from build123d import *

# Parameters (mm, degrees)
F1_DEPTH = 23
F3_DEPTH = 21
F4_R     = 12.5
F4_R_2   = 1.75
F5_DEPTH = 22.001


with BuildPart() as f1:
    # F0 (on Right) → F1 (new body, symmetric)
    with BuildSketch(Plane.YZ):
        Polygon((2, 44), (0, 44), (0, 0), (22, 0), (22, 2), align=None)
    extrude(amount=F1_DEPTH, both=True)

    # F2 (on Right) → F3 (cut, symmetric)
    with BuildSketch(Plane.YZ):
        Polygon((2, 2), (22, 2), (2, 44), align=None)
    extrude(amount=F3_DEPTH, both=True, mode=Mode.SUBTRACT)

    # F4 (on face) → F5 (cut, through all)
    with BuildSketch(Plane.XZ):
        with Locations((0, 23)):
            Circle(F4_R)
        with Locations((-15.5, 38.5)):
            Circle(F4_R_2)
        with Locations((-15.5, 7.5)):
            Circle(F4_R_2)
        with Locations((15.5, 38.5)):
            Circle(F4_R_2)
        with Locations((15.5, 7.5)):
            Circle(F4_R_2)
    extrude(amount=-F5_DEPTH, mode=Mode.SUBTRACT)


solid = f1.part
Input: part model. Units: mm. Frame: model coordinates. A direction names the side the tool comes from. Give positions to 0.01 mm unless a question says otherwise; leave off trailing zeros. Loops run counter-clockwise (first coordinate to the right, second up) from the corner with the lowest first, then second, coordinate; pieces in that order, holes last. Notation, with made-up numbers: (4, 12) -> (27, 12) arc R19 cw to (27, 39) -> close; hole circle Ø10 at (-14, -30). An arc over 180 degrees is marked (long way). Answer as a JSON object with one key per item and string values. Group by question number.
Item 1: Pull-direction query (X, two-part tool) for faces 3 (the flat face through (-22, 12, 23)), 4 (the flat face through (23, 8, 17)), 5 (the flat face through (0, 12, 2)); classes: released by +X, released by -X, zero draft, split by the parting line, or undercut.
Item 2: Cut plane D-D, the plane z = 26. Return the cut outline in (x, y), and give its area (3 significant figures).
Item 3: Cut plane B-B, the plane z = 38.5. Return the cut outline in (x, y), and give its area (3 significant figures).
Item 4: Cut plane C-C, the plane y = 16. Return the cut outline in (x, z).
Item 5: Cut plane A-A, the plane x = 0. Return the cut outline in (y, z), and give its area (3 significant figures).
Item 6: Reachability of faces 1 (the flat face through (21, 7, 14)), 2 (the flat face through (-10, 0, 13)) from +Z, -Z, +X, -X, +Y, -Y: full face, straight path, thin tool, end or side. Return the list, or none.
Item 7: Line query: probe 1 along Z at (x, y) = (15.5, 0.5); probe 2 along X at (y, z) = (11.5, 20.5); probe 3 along Z at (x, y) = (-4, 4.25). Output: solid intervals per line, ascending.
Item 8: Pin query (flat end, axial travel): P1, Ø3, axis at x = -14, z = 23.5, coming from the +Y side. Return the tip coordinate at first contact, or that it passes through.
Checks:
{
 "1": {"face 3": "zero draft", "face 4": "released by +X", "face 5": "undercut"},
 "2": {"outline": "(-23, 0) -> (-12.13, 0) -> (-12.13, 2) -> (-21, 2) -> (-21, 10.57) -> (-23, 10.57) -> close; (12.13, 0) -> (23, 0) -> (23, 10.57) -> (21, 10.57) -> (21, 2) -> (12.13, 2) -> close", "area": "77.7 mm²"},
 "3": {"outline": "(-23, 0) -> (-17.25, 0) -> (-17.25, 2) -> (-21, 2) -> (-21, 4.62) -> (-23, 4.62) -> close; (-13.75, 0) -> (13.75, 0) -> (13.75, 2) -> (-13.75, 2) -> close; (17.25, 0) -> (23, 0) -> (23, 4.62) -> (21, 4.62) -> (21, 2) -> (17.25, 2) -> close", "area": "88.5 mm²"},
 "4": {"outline": "(-23, 0) -> (23, 0) -> (23, 14.6) -> (21, 14.6) -> (21, 2) -> (-21, 2) -> (-21, 14.6) -> (-23, 14.6) -> close"},
 "5": {"outline": "(0, 0) -> (22, 0) -> (22, 2) -> (2, 2) -> (2, 10.5) -> (0, 10.5) -> close; (0, 35.5) -> (2, 35.5) -> (2, 44) -> (0, 44) -> close", "area": "78.0 mm²"},
 "6": {"face 1": "+Z, +Y", "face 2": "+Z, -Z, +X, -X, -Y"},
 "7": {"probe 1": "z = 0 to 5.75, 9.25 to 36.75, 40.25 to 44", "probe 2": "x = -23 to -21, 21 to 23", "probe 3": "z = 0 to 2"},
 "8": {"P1": "stops at y = 2"}
}
